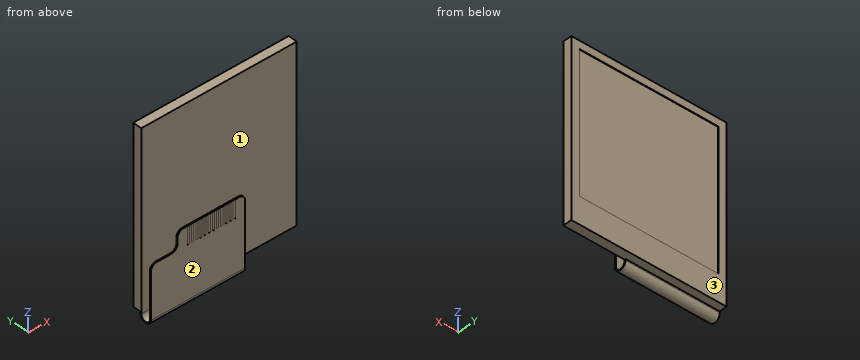
from build123d import *

# Parameters (mm, degrees)
SKETCH_1_W          = 26.16
SKETCH_1_H          = 29.22
EXTRUDE_1_DEPTH     = 1.5
EXTRUDE_2_DEPTH     = 15.86
SKETCH_4_W          = 4.46
SKETCH_4_H          = 3
CUT_EXTRUDE_1_DEPTH = 1
FILLET_2_R          = 1
SKETCH_5_W          = 23.4
SKETCH_5_H          = 23.4
CUT_EXTRUDE_2_DEPTH = 0.1
SKETCH_6_W          = 0.35
SKETCH_6_H          = 3
CUT_EXTRUDE_3_DEPTH = 0.005


with BuildPart() as part:
    # 草图1 → 凸台-拉伸1 (new body)
    with BuildSketch(Plane(origin=(0, 0, 0), x_dir=(1, 0, 0), z_dir=(0, 1, 0))):
        Rectangle(SKETCH_1_W, SKETCH_1_H)
    extrude(amount=EXTRUDE_1_DEPTH)

    # 草图3 → 凸台-拉伸2 (add)
    with BuildSketch(Plane.ZY.offset(13.08)):
        with BuildLine():
            Line((-14.61, 0), (-14.864156079, 0))
            ThreePointArc((-14.864156079, 0), (-15.664156079, -0.8), (-14.864156079, -1.6))
            Line((-14.864156079, -1.6), (-3.11, -1.6))
            Line((-3.11, -1.6), (-3.11, -1.8))
            Line((-3.11, -1.8), (-14.864156079, -1.8))
            ThreePointArc((-14.864156079, -1.8), (-15.864156079, -0.8), (-14.864156079, 0.2))
            Line((-14.864156079, 0.2), (-14.61, 0.2))
            Line((-14.61, 0.2), (-14.61, 0))
        make_face()
    extrude(amount=-EXTRUDE_2_DEPTH)

    # 草图4 → 切除-拉伸1 (cut)
    with BuildSketch(Plane.XZ.offset(1.8)):
        with Locations((-10.85, -4.61)):
            Rectangle(SKETCH_4_W, SKETCH_4_H)
    extrude(amount=-CUT_EXTRUDE_1_DEPTH, mode=Mode.SUBTRACT)

    # 圆角2
    fillet_2_edges = [part.edges().sort_by_distance(p)[0] for p in [
        (2.78, -1.7, -3.11),
        (-13.08, -1.7, -6.11),
        (-8.62, -1.7, -3.11),
        (-8.62, -1.7, -6.11),
    ]]
    fillet(fillet_2_edges, radius=FILLET_2_R)

    # 草图5 → 切除-拉伸2 (cut)
    with BuildSketch(Plane(origin=(0, 1.5, 0), x_dir=(1, 0, 0), z_dir=(0, 1, 0))):
        with Locations((0, -1.58)):
            Rectangle(SKETCH_5_W, SKETCH_5_H)
    extrude(amount=-CUT_EXTRUDE_2_DEPTH, mode=Mode.SUBTRACT)

    # 草图6 → 切除-拉伸3 (cut)
    with BuildSketch(Plane.XZ.offset(1.8)):
        with Locations((-6.765, -4.61)):
            Rectangle(SKETCH_6_W, SKETCH_6_H)
        with Locations((-6.065, -4.61)):
            Rectangle(SKETCH_6_W, SKETCH_6_H)
        with Locations((-5.365, -4.61)):
            Rectangle(SKETCH_6_W, SKETCH_6_H)
        with Locations((-4.665, -4.61)):
            Rectangle(SKETCH_6_W, SKETCH_6_H)
        with Locations((-3.965, -4.61)):
            Rectangle(SKETCH_6_W, SKETCH_6_H)
        with Locations((-3.265, -4.61)):
            Rectangle(SKETCH_6_W, SKETCH_6_H)
        with Locations((-2.565, -4.61)):
            Rectangle(SKETCH_6_W, SKETCH_6_H)
        with Locations((-1.865, -4.61)):
            Rectangle(SKETCH_6_W, SKETCH_6_H)
        with Locations((-1.165, -4.61)):
            Rectangle(SKETCH_6_W, SKETCH_6_H)
        with Locations((-0.465, -4.61)):
            Rectangle(SKETCH_6_W, SKETCH_6_H)
        with Locations((0.235, -4.61)):
            Rectangle(SKETCH_6_W, SKETCH_6_H)
        with Locations((0.935, -4.61)):
            Rectangle(SKETCH_6_W, SKETCH_6_H)
    extrude(amount=-CUT_EXTRUDE_3_DEPTH, mode=Mode.SUBTRACT)


solid = part.part
The model under review builds one solid part; all positions refer to its coordinate system, in mm. Face numbers are marked on the shaded views. Round coordinates to 2 decimals unless told otherwise and drop trailing zeros. Loops run counter-clockwise (first coordinate to the right, second up) from the corner with the lowest first, then second, coordinate; pieces in that order, holes last. Notation, with made-up numbers: M 42.5,-20.75 L 59.5,-20.75 A20 ccw 59.5,17.25 Z; hole C 19,82.5 d8. An arc over 180 degrees is marked long. Answer as CSV lines item,"result". Start each with the question number.
Item 1: Wall thickness on line 1 (Y direction, x = 2.5, z = -9); line 2 (Y direction, x = -4.5, z = -11); line 3 (Y direction, x = -7.75, z = -2): over which ranges is each line inside the solid? List them lowest first. Write a range as [from, to].
Item 2: Consider section C-C (z = -6.5). Write out the cut boundary in (x, y).
Item 3: Consider section B-B (x = 9.5). Write out the cut boundary in (y, z).
Item 4: Consider section D-D (y = -0.8). Write out the cut boundary in (x, z).
Item 5: Consider section A-A (z = 11). Write out the cut boundary in (x, y), then the cut area to 3 significant figures.
Item 6: Insertion check: P1, Ø8, axis at x = 3, z = 11, coming from the -Y side; P2, Ø1, axis at x = 7, y = -1, coming from the +Z side. Each pin has a flat end and moves straight along its axis. Give the tip position at first contact, or say it passes through.
Item 7: Mouldability with a two-part tool opening along Y and no side actions: class the marked faces 1, 2 and 3 as released by +Y, released by -Y, zero draft, split by the parting line, or undercut.
Answer:
1,line 1,"y = [-1.8, -1.6], [0, 1.4]"
1,line 2,"y = [-1.8, -1.6], [0, 1.5]"
1,line 3,"y = [0, 1.4]"
2,outline,"M -13.08,0 L 13.08,0 L 13.08,1.5 L 11.7,1.5 L 11.7,1.4 L -11.7,1.4 L -11.7,1.5 L -13.08,1.5 Z; M -12.87,-1.8 L 2.78,-1.8 L 2.78,-1.6 L -12.87,-1.6 Z"
3,outline,"M 0,-14.61 L 1.5,-14.61 L 1.5,-10.12 L 1.4,-10.12 L 1.4,13.28 L 1.5,13.28 L 1.5,14.61 L 0,14.61 Z"
4,outline,"M -13.08,-15.86 L 2.78,-15.86 L 2.78,-15.66 L -13.08,-15.66 Z"
5,outline,"M -13.08,0 L 13.08,0 L 13.08,1.5 L 11.7,1.5 L 11.7,1.4 L -11.7,1.4 L -11.7,1.5 L -13.08,1.5 Z"
5,area,"36.9 mm^2"
6,P1,"stops at y = 0"
6,P2,"passes through"
7,face 1,"undercut"
7,face 2,"released by -Y"
7,face 3,"released by +Y"
